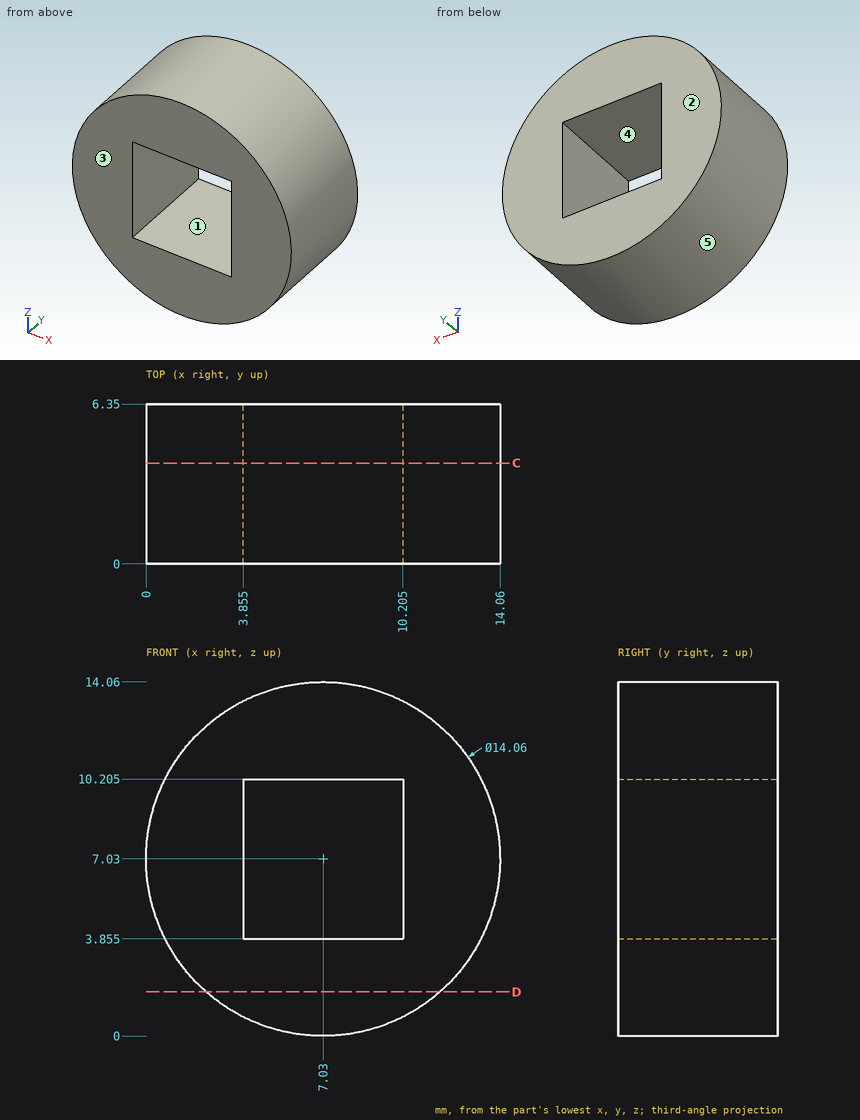
Here's the drawing with two shaded views (mm, measured from the low corner). I have some questions. A direction names the side the tool comes from. Coordinates: 2 decimals unless noted, no trailing zeros. Order: outer loops, then holes, each group sorted by start corner. A loop starts at its lowest first (then second) coordinate and runs counter-clockwise, first axis right, second up. Notation, with made-up numbers: (-38.5, -13) -> (-23.5, -13) arc R17 cw to (-23.5, -2) -> close; hole circle Ø5 at (80, 28). An arc over 180 degrees is marked (long way). Write each question's results on one line, items separated by ' | '.
Item 1: I'm going to push flat-ended pins straight in: pin 1 Ø1.9 at (x, y) = (7.5, 4.5) entering from +Z; pin 2 Ø1 at (x, y) = (9.5, 3) entering from +Z. Where does each tip first touch, or does it pass through?
Results are:
pin 1: z = 14.06 | pin 2: z = 13.78
Item 2: If I drill on line 1 along Z through (x, y) = (7, 1.75) (1 decimal); line 2 along X through (y, z) = (3.5, 8.25) (1 decimal); line 3 along Z through (x, y) = (9, 6) (1 decimal), over which ranges is the centre line in solid material (lowest first)?
Results are:
line 1: 0 to 3.9, 10.2 to 14.1 | line 2: 0.1 to 3.9, 10.2 to 14 | line 3: 0.3 to 3.9, 10.2 to 13.8
Item 3: Which directions (+Z, -Z, +X, -X, +Y, -Y) give clear straight access to the entire face, cutting with the end or side of a thin tool? Please do the marked faces 1 and 2.
Results are:
face 1: +Y, -Y | face 2: +Z, -Z, +X, -X, +Y
Item 4: If we mould it in two halves opening along X, with no side actions, what happens to the marked faces 3, 4 and 5? For each: +X half, -X half, draft (parallel to the pull), parting line (faces both ways), or undercut.
Results are:
face 3: draft | face 4: undercut | face 5: parting line
Item 5: I want a section at C-C, the plane y = 4. Write out the boundary of the cut face in (x, z) (1 decimal).
Results are:
outline: circle Ø14.1 at (7, 7); hole (3.9, 3.9) -> (10.2, 3.9) -> (10.2, 10.2) -> (3.9, 10.2) -> close
Item 6: I want a section at D-D, the plane z = 1.75. Write out the boundary of the cut face in (x, y).
Results are:
outline: (2.39, 0) -> (11.67, 0) -> (11.67, 6.35) -> (2.39, 6.35) -> close
